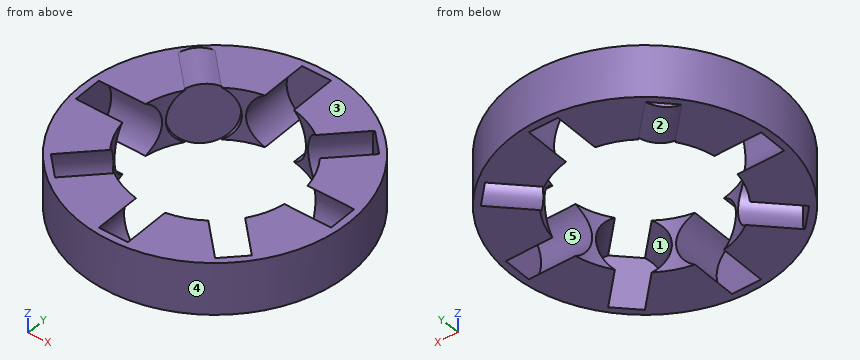
```python
from build123d import *

# Parameters (mm, degrees)
SKETCH1_R                   = 18
SKETCH1_R_2                 = 11
BOSS_EXTRUDE1_DEPTH         = 3.5
SKETCH4_R                   = 4
CUT_EXTRUDE1_DEPTH          = 6.9
CIRPATTERN1_COUNT           = 8
SKETCH5_R                   = 4
SPACECLAIM_FOR_MAGNET_DEPTH = 6


with BuildPart() as part:
    # Sketch1 → Boss-Extrude1 (new body, symmetric)
    with BuildSketch(Plane.XY):
        Circle(SKETCH1_R)
        Circle(SKETCH1_R_2, mode=Mode.SUBTRACT)
    extrude(amount=BOSS_EXTRUDE1_DEPTH, both=True)

    # Sketch4 → Cut-Extrude1 (cut)
    with BuildSketch(Plane(origin=(-10.162674858, 0, 0), x_dir=(0, 0, -1), z_dir=(1, 0, 0))):
        Circle(SKETCH4_R)
    cut_extrude1 = extrude(amount=-CUT_EXTRUDE1_DEPTH, mode=Mode.SUBTRACT)

    # CirPattern1: Cut-Extrude1 ×8 about axis
    cirpattern1_axis = Axis((0, 0, 0), (0, 0, 1))
    for i in range(1, CIRPATTERN1_COUNT):
        add(cut_extrude1.rotate(cirpattern1_axis, i * 360 / CIRPATTERN1_COUNT), mode=Mode.SUBTRACT)

    # Sketch5 → SpaceClaim for Magnet (add)
    with BuildSketch(Plane(origin=(-12.065133097, 12.065133097, 0), x_dir=(0.707106781, 0.707106781, 0), z_dir=(0.707106781, -0.707106781, 0))):
        Circle(SKETCH5_R)
    extrude(amount=SPACECLAIM_FOR_MAGNET_DEPTH)


solid = part.part
```
Part model, mm, in its own coordinate system. Face numbers are marked on the shaded views. A direction names the side the tool comes from. Give positions to 0.01 mm unless a question says otherwise; leave off trailing zeros. Write each loop counter-clockwise with the first axis right and the second up, starting at its lowest first coordinate (ties: lowest second). Pieces come first, ordered by that corner, then holes. Notation, with made-up numbers: (16.25, 47.25) -> (65.25, 47.25) arc R30 cw to (65.25, 83.25) -> close; hole circle Ø9 at (25.5, 12.5). An arc over 180 degrees is marked (long way). Put each result on its own line as item: value. Start each with the question number.
Item 1: Pull direction Z, two halves, no side cores. Call the marked faces 1, 2 and 3: pulls with the +Z half, pulls with the -Z half, needs draft (parallel to the pull), parting line crosses it, or undercut.
Item 2: Wall check: L1, parallel to X at y = 11.5, z = -2.25; L2, parallel to Y at x = 11, z = 0.25; L3, parallel to Y at x = -10.5, z = 0.5. Give the ranges that are in metal, low to high. Write a range as [from, to].
Item 3: Pin check, flat tips, straight feed: pin 1 Ø18 at (x, y) = (7, -1) entering from -Z; pin 2 Ø1.5 at (x, z) = (10.5, -3) entering from -Y; pin 3 Ø1.5 at (x, z) = (3.5, -1) entering from -Y. Stop position of each tip, or through.
Item 4: Which spindle directions (+Z, -Z, +X, -X, +Y, -Y) get a long thin tool onto all of the face, cutting with end or side? Do the marked faces 4 and 5. Say none if no direction does.
Item 5: Cut at A-A (y = 0). List the corners of the cut face in (x, z), then the cut area to 3 significant figures.
Answer list:
1. face 1: undercut
1. face 2: pulls with the -Z half
1. face 3: pulls with the +Z half
2. L1: x = [-13.85, -3.31], [3.31, 6.82], [12.63, 13.85]
2. L2: y = [-14.25, -13.13], [-5.35, -3.99], [3.99, 5.35], [13.13, 14.25]
2. L3: y = [-14.62, -13.63], [-4.89, -3.97], [3.97, 4.89], [5.14, 14.62]
3. pin 1: stops at z = -3.5
3. pin 2: stops at y = -15.13
3. pin 3: stops at y = -17.79
4. face 4: +Z, -Z
4. face 5: none
5. outline: (-18, -3.5) -> (-17.06, -3.5) -> (-17.06, 3.5) -> (-18, 3.5) -> close; (17.06, -3.5) -> (18, -3.5) -> (18, 3.5) -> (17.06, 3.5) -> close
5. area: 13.1 mm2
